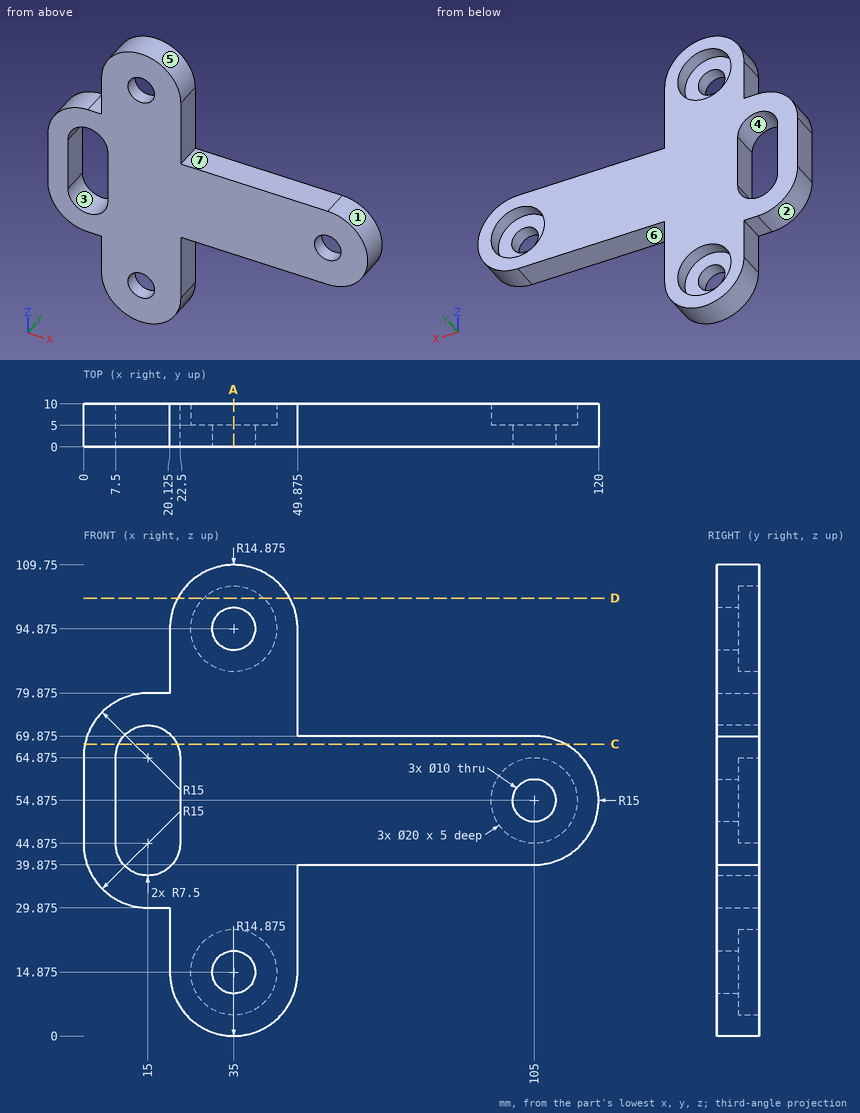
Study the drawing (mm; zero at the part's minimum x, y, z) and answer. A direction names the side the tool comes from. Round coordinates to 2 decimals unless told otherwise and drop trailing zeros. Order: outer loops, then holes, each group sorted by start corner. A loop starts at its lowest first (then second) coordinate and runs counter-clockwise, first axis right, second up. Notation, with made-up numbers: M 49,24.25 L 88,24.25 A30 ccw 88,49.25 Z; hole C 76.5,37 d2. An arc over 180 degrees is marked long. One line per item, written item: value.
Q1. Flat-ended cylindrical pins translate along their axes: pin 1 (22 mm diameter, centred on x = 38, z = 94, fed in from +Y); pin 2 (11.5 mm diameter, centred on x = 35, z = 14.88, fed in from +Y); pin 3 (1 mm diameter, centred on y = 8.5, z = 53, fed in from +X); pin 4 (1 mm diameter, centred on x = 66.5, y = 5, fed in from -Z) (1 decimal). Find the tip coordinate at first contact, or state that the pin passes through.
Derived:
pin 1: y = 10
pin 2: y = 5
pin 3: x = 119.94
pin 4: z = 39.9
Q2. For the marked faces 5, 6 and 7, determine the directions among +Z, -Z, +X, -X, +Y, -Y from which every point of the face is accessible in a straight line to the end or side of a thin tool.
Derived:
face 5: +Z, +Y, -Y
face 6: -Z, +X, +Y, -Y
face 7: +Z, +X, +Y, -Y
Q3. Determine the mould class of the marked faces 1, 2, 3 and 4 for opening direction Z: released by +Z, released by -Z, zero draft, split by the parting line, or undercut.
Derived:
face 1: split by the parting line
face 2: released by -Z
face 3: undercut
face 4: undercut
Q4. Straight lines are drawn through the part: line 1 (Z direction, x = 51, y = 2.5) (1 decimal); line 2 (X direction, y = 4.75, z = 38) (1 decimal); line 3 (Y direction, x = 31.5, z = 87). For each, find the intervals that lie inside material, in ascending order.
Derived:
line 1: 39.9 to 69.9
line 2: 1.7 to 12, 18 to 49.9
line 3: 0 to 5
Q5. Find section C-C on z = 68. Write down the section's boundary in (x, y), then the cut area to 3 significant figures.
Derived:
outline: M 0.33,0 L 8.18,0 L 8.18,10 L 0.33,10 Z; M 21.82,0 L 112.26,0 L 112.26,10 L 21.82,10 Z
area: 983 mm²
Q6. Find section D-D on z = 102. Write down the section's boundary in (x, y), then the cut area to 3 significant figures.
Derived:
outline: M 21.94,0 L 48.06,0 L 48.06,10 L 42.02,10 L 42.02,5 L 27.98,5 L 27.98,10 L 21.94,10 Z
area: 191 mm²
Q7. Find section A-A on x = 35. Give the number of separate pieces and of enclosed holes in the cut face.
Derived:
separate pieces: 3
enclosed holes: 0
